Design review of the part built by this model. Coordinates are the model's own, in mm. A direction names the side the tool comes from. Round coordinates to 2 decimals unless told otherwise and drop trailing zeros. Loops run counter-clockwise (first coordinate to the right, second up) from the corner with the lowest first, then second, coordinate; pieces in that order, holes last. Notation, with made-up numbers: (74.25, 86) -> (102.25, 86) arc R17 ccw to (102.25, 111) -> close; hole circle Ø3 at (1.5, -36.75). An arc over 180 degrees is marked (long way). Use a Markdown table: item, result. Add a question column.
from build123d import *

# Parameters (mm, degrees)
SKETCH1_W           = 50
SKETCH1_H           = 16
BOSS_EXTRUDE1_DEPTH = 10
SKETCH2_R           = 2.75
CUT_EXTRUDE1_DEPTH  = 29.08914381
SKETCH3_R           = 2.5
BOSS_EXTRUDE2_DEPTH = 8
FILLET1_R           = 0.5
SKETCH4_W           = 50
SKETCH4_H           = 10
CUT_EXTRUDE2_DEPTH  = 2
SKETCH5_W           = 50
SKETCH5_H           = 10
BOSS_EXTRUDE3_DEPTH = 2.9
BOSS_EXTRUDE4_DEPTH = 50
FILLET2_R           = 2
SKETCH7_R           = 4.5
CUT_EXTRUDE3_DEPTH  = 3
CHAMFER1_SIZE       = 0.5


with BuildPart() as part:
    # Sketch1 → Boss-Extrude1 (new body)
    with BuildSketch(Plane.XY):
        Rectangle(SKETCH1_W, SKETCH1_H)
    extrude(amount=BOSS_EXTRUDE1_DEPTH)

    # Sketch2 → Cut-Extrude1 (cut, through all)
    with BuildSketch(Plane.XY.offset(10)):
        Circle(SKETCH2_R)
    extrude(amount=-CUT_EXTRUDE1_DEPTH, mode=Mode.SUBTRACT)

    # Sketch3 → Boss-Extrude2 (add)
    with BuildSketch(Plane.XY.offset(10)):
        with Locations((-16, 0)):
            Circle(SKETCH3_R)
        with Locations((16, 0)):
            Circle(SKETCH3_R)
    extrude(amount=BOSS_EXTRUDE2_DEPTH)

    # Fillet1
    fillet1_edges = [part.edges().sort_by_distance(p)[0] for p in [
        (-18.5, 0, 18),
        (13.5, 0, 18),
    ]]
    fillet(fillet1_edges, radius=FILLET1_R)

    # Sketch4 → Cut-Extrude2 (cut)
    with BuildSketch(Plane(origin=(0, -8, 0), x_dir=(-1, 0, 0), z_dir=(0, -1, 0))):
        with Locations((0, -5)):
            Rectangle(SKETCH4_W, SKETCH4_H)
    extrude(amount=-CUT_EXTRUDE2_DEPTH, mode=Mode.SUBTRACT)

    # Sketch5 → Boss-Extrude3 (add)
    with BuildSketch(Plane(origin=(0, 8, 0), x_dir=(1, 0, 0), z_dir=(0, 1, 0))):
        with Locations((0, -5)):
            Rectangle(SKETCH5_W, SKETCH5_H)
    extrude(amount=BOSS_EXTRUDE3_DEPTH)

    # Sketch6 → Boss-Extrude4 (add, through all)
    with BuildSketch(Plane(origin=(25, 0, 0), x_dir=(0, 0, -1), z_dir=(1, 0, 0))):
        Polygon((-14.1, 10.9), (-10, 6.8), (-10, 10.9), align=None)
    extrude(amount=-BOSS_EXTRUDE4_DEPTH)

    # Fillet2
    fillet2_edges = [part.edges().sort_by_distance(p)[0] for p in [
        (25, 2.45, 0),
        (0, 10.9, 0),
        (-25, 2.45, 0),
    ]]
    fillet(fillet2_edges, radius=FILLET2_R)

    # Sketch7 → Cut-Extrude3 (cut)
    with BuildSketch(Plane.XY.offset(10)):
        Circle(SKETCH7_R)
    extrude(amount=-CUT_EXTRUDE3_DEPTH, mode=Mode.SUBTRACT)

    # Chamfer1
    chamfer1_edges = [part.edges().sort_by_distance(p)[0] for p in [
        (-4.5, 0, 10),
    ]]
    chamfer(chamfer1_edges, length=CHAMFER1_SIZE)


solid = part.part
1. Mouldability with a two-part tool opening along X and no side actions: class faces 4 (the face through (0, 10.9, 8)), 5 (the face through (-24.43, 2.33, 0.6)), 6 (the face through (-18.5, 0.1, 13.7)) as +X half, -X half, draft (parallel to the pull), parting line (faces both ways), or undercut.
2. Consider section B-B on x = 0. State the section outline as (y, z) points.
3. Consider section C-C on z = 4.25. State the section outline as (x, y) points, plus the area to 3 significant figures.
4. For faces 1 (the face through (-0.59, 4.46, 8.27)), 2 (the face through (0, 3, 0)), 3 (the face through (0.4, 8.9, 12.1)), list the 3-axis set-ups (+Z, -Z, +X, -X, +Y, -Y) from which the entire face can be reached by the end or side of a thin tool; tool diameter is ignored.
5. Consider section A-A on y = 0. State the section outline as (x, z) points, plus the area to 3 significant figures.
6. Consider section D-D on x = -16. State the section outline as (y, z) points.
7. To check wall thickness, follow probe 1 along Y at (x, z) = (0, 4); probe 2 along Y at (x, z) = (0, 8.35); probe 3 along X at (y, z) = (1.5, 13). State the ranges of each line that lie inside material, in increasing order. Write a range as from..to.
8. Insertion check: P1, Ø1.5, axis at x = 10, y = -0.5, coming from the +Z side; P2, Ø5, axis at x = 0, y = 0, coming from the +Z side; P3, Ø10, axis at x = -11.5, y = 0.5, coming from the +Z side; P4, Ø6, axis at x = -5, y = 6.5, coming from the +Z side. Each pin has a flat end and moves straight along its axis. Give the tip position at first contact, or say it passes through.
Verdict:
| question | item | result |
|---|---|---|
| 1 | face 4 | draft |
| 1 | face 5 | -X half |
| 1 | face 6 | undercut |
| 2 | outline | (-6, 0) -> (-2.75, 0) -> (-2.75, 7) -> (-4.5, 7) -> (-4.5, 9.5) -> (-5, 10) -> (-6, 10) -> close; (2.75, 0) -> (8.9, 0) arc R2 ccw to (10.9, 2) -> (10.9, 14.1) -> (6.8, 10) -> (5, 10) -> (4.5, 9.5) -> (4.5, 7) -> (2.75, 7) -> close |
| 3 | outline | (-25, -6) -> (25, -6) -> (25, 10.9) -> (-25, 10.9) -> close; hole circle Ø5.5 at (0, 0) |
| 3 | area | 821 mm² |
| 4 | face 1 | +Z |
| 4 | face 2 | -Z, +X, -X, +Y, -Y |
| 4 | face 3 | +Z, +X, -X |
| 5 | outline | (-25, 2) arc R2 ccw to (-23, 0) -> (-2.75, 0) -> (-2.75, 7) -> (-4.5, 7) -> (-4.5, 9.5) -> (-5, 10) -> (-13.5, 10) -> (-13.5, 17.5) arc R0.5 ccw to (-14, 18) -> (-18, 18) arc R0.5 ccw to (-18.5, 17.5) -> (-18.5, 10) -> (-25, 10) -> close; (2.75, 0) -> (23, 0) arc R2 ccw to (25, 2) -> (25, 10) -> (18.5, 10) -> (18.5, 17.5) arc R0.5 ccw to (18, 18) -> (14, 18) arc R0.5 ccw to (13.5, 17.5) -> (13.5, 10) -> (5, 10) -> (4.5, 9.5) -> (4.5, 7) -> (2.75, 7) -> close |
| 5 | area | 512 mm² |
| 6 | outline | (-6, 0) -> (8.9, 0) arc R2 ccw to (10.9, 2) -> (10.9, 14.1) -> (6.8, 10) -> (2.5, 10) -> (2.5, 17.5) arc R0.5 ccw to (2, 18) -> (-2, 18) arc R0.5 ccw to (-2.5, 17.5) -> (-2.5, 10) -> (-6, 10) -> close |
| 7 | probe 1 | y = -6..-2.75, 2.75..10.9 |
| 7 | probe 2 | y = -6..-4.5, 4.5..10.9 |
| 7 | probe 3 | x = -18..-14, 14..18 |
| 8 | P1 | stops at z = 10 |
| 8 | P2 | passes through |
| 8 | P3 | stops at z = 18 |
| 8 | P4 | stops at z = 12.7 |
